Geometry check sheet. Reference: the model listing, model coordinates, mm. Coordinates: 2 decimals unless noted, no trailing zeros. Order: outer loops, then holes, each group sorted by start corner. A loop starts at its lowest first (then second) coordinate and runs counter-clockwise, first axis right, second up. Notation, with made-up numbers: M 16.25,-5.5 L 68.25,-5.5 A10 ccw 68.25,3.5 Z; hole C -34,-37 d6. An arc over 180 degrees is marked long. Use CSV: the item, a comma, the result in double quotes. Start each with the question number.
```python
from build123d import *

# Parameters (mm, degrees)
BOSS_EXTRUDE1_DEPTH = 25.4


with BuildPart() as part:
    # Sketch1 → Boss-Extrude1 (new body)
    with BuildSketch(Plane.XY):
        with BuildLine():
            ThreePointArc((0, 25.4), (-12.7, 12.7), (0, 0))
            Line((0, 0), (0, 25.4))
        make_face()
        with BuildLine():
            Line((0, 25.4), (0, 0))
            ThreePointArc((0, 0), (8.980256121, 3.719743879), (12.7, 12.7))
            ThreePointArc((12.7, 12.7), (8.980256121, 21.680256121), (0, 25.4))
        make_face()
        with BuildLine():
            ThreePointArc((12.7, 12.7), (8.980256121, 3.719743879), (0, 0))
            Line((0, 0), (177.8, 0))
            ThreePointArc((177.8, 0), (165.1, 12.7), (177.8, 25.4))
            Line((177.8, 25.4), (0, 25.4))
            ThreePointArc((0, 25.4), (8.980256121, 21.680256121), (12.7, 12.7))
        make_face()
        with BuildLine():
            ThreePointArc((177.8, 25.4), (165.1, 12.7), (177.8, 0))
            Line((177.8, 0), (177.8, 25.4))
        make_face()
        with BuildLine():
            Line((177.8, 25.4), (177.8, 0))
            ThreePointArc((177.8, 0), (186.780256121, 3.719743879), (190.5, 12.7))
            ThreePointArc((190.5, 12.7), (186.780256121, 21.680256121), (177.8, 25.4))
        make_face()
    extrude(amount=BOSS_EXTRUDE1_DEPTH)


solid = part.part
```
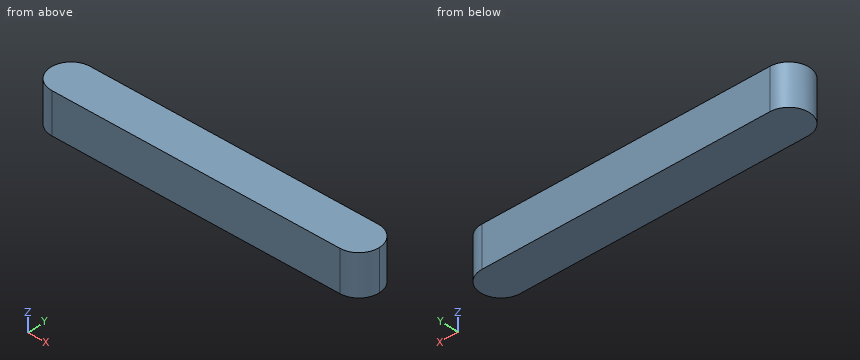
1) Section check B-B on y = 22. Record the boundary of the cut face in (x, z).
2) Material ranges on line 1 along X through (y, z) = (16.5, 24.25); line 2 along X through (y, z) = (5.75, 1.75); line 3 along Y through (x, z) = (181, 6.5), recorded low to high.
3) Section check C-C on y = 2.5. Record the boundary of the cut face in (x, z).
4) Section check A-A on z = 4.75. Record the boundary of the cut face in (x, y), then the cut area to 3 significant figures.
5) Gauge pin test, flat ends, axial feed: P1, Ø10, axis at y = 6.5, z = 16.5, coming from the +X side; P2, Ø1.5, axis at y = 11, z = 4, coming from the -X side; P3, Ø4, axis at y = 10, z = 18, coming from the +X side. Record the tip position at first contact, or that the pin passes through.
Results are:
1,outline,"M -8.65,0 L 186.45,0 L 186.45,25.4 L -8.65,25.4 Z"
2,line 1,"x = -12.12 to 189.92"
2,line 2,"x = -10.63 to 188.43"
2,line 3,"y = 0.41 to 24.99"
3,outline,"M -7.57,0 L 185.37,0 L 185.37,25.4 L -7.57,25.4 Z"
4,outline,"M 0,0 L 177.8,0 A12.7 ccw 177.8,25.4 L 0,25.4 A12.7 ccw Z"
4,area,"5,020 mm²"
5,P1,"stops at x = 190.44"
5,P2,"stops at x = -12.66"
5,P3,"stops at x = 190.48"
